The model under review builds one solid part; all positions refer to its coordinate system, in mm. Coordinates: 2 decimals unless noted, no trailing zeros. Write each loop counter-clockwise with the first axis right and the second up, starting at its lowest first coordinate (ties: lowest second). Pieces come first, ordered by that corner, then holes. Notation, with made-up numbers: (38.25, -33) - (45.25, -33) arc R14 cw to (45.25, -29) - close; hole circle Ø6 at (-23.75, -10.5). An arc over 180 degrees is marked (long way). Put each result on its own line as item: value.
from build123d import *

# Parameters (mm, degrees)
BOSS_EXTRUDE1_DEPTH = 914.4
SKETCH2_R           = 6.35
CUT_EXTRUDE1_DEPTH  = 153.4


with BuildPart() as part:
    # Sketch1 → Boss-Extrude1 (new body, symmetric)
    with BuildSketch(Plane.XY):
        with BuildLine():
            Line((0, 0), (0, 152.4))
            Line((0, 152.4), (0.00508, 152.4))
            ThreePointArc((0.00508, 152.4), (6.736679988, 149.611679988), (9.525, 142.88008))
            Line((9.525, 142.88008), (9.525, 22.225))
            ThreePointArc((9.525, 22.225), (13.244743879, 13.244743879), (22.225, 9.525))
            Line((22.225, 9.525), (41.28008, 9.525))
            ThreePointArc((41.28008, 9.525), (48.011679988, 6.736679988), (50.8, 0.00508))
            Line((50.8, 0.00508), (50.8, 0))
            Line((50.8, 0), (0, 0))
        make_face()
    extrude(amount=BOSS_EXTRUDE1_DEPTH, both=True)

    # Sketch2 → Cut-Extrude1 (cut, through all)
    with BuildSketch(Plane.XZ):
        with Locations((25.4, -711.2)):
            Circle(SKETCH2_R)
        with Locations((25.4, -203.2)):
            Circle(SKETCH2_R)
        with Locations((25.4, 203.2)):
            Circle(SKETCH2_R)
        with Locations((25.4, 711.2)):
            Circle(SKETCH2_R)
    extrude(amount=-CUT_EXTRUDE1_DEPTH, mode=Mode.SUBTRACT)


solid = part.part
1. For pin 1 Ø3 at (x, z) = (25, -299) entering from +Y (3 decimals); pin 2 Ø3 at (y, z) = (127, 297.5) entering from +X (3 decimals), all flat-tipped, find the tip position at first contact; note any pin that passes through.
Determined:
pin 1: stops at y = 9.525
pin 2: stops at x = 9.525
2. To check wall thickness, follow probe 1 along Z at (x, y) = (25.4, 5); probe 2 along Y at (x, z) = (22, -556.5); probe 3 along X at (y, z) = (140.5, -86.5) (3 decimals). State the ranges of each line that lie inside material, in increasing order.
Determined:
probe 1: z = -914.4 to -717.55, -704.85 to -209.55, -196.85 to 196.85, 209.55 to 704.85, 717.55 to 914.4
probe 2: y = 0 to 9.53
probe 3: x = 0 to 9.525
3. Consider section B-B on y = 100.5. State the section outline as (x, z) points (3 decimals).
Determined:
outline: (0, -914.4) - (9.525, -914.4) - (9.525, 914.4) - (0, 914.4) - close
4. Consider section A-A on z = 75. State the section outline as (x, y) points (3 decimals), plus the area to 3 significant figures.
Determined:
outline: (0, 0) - (50.8, 0) - (50.8, 0.005) arc R9.52 ccw to (41.28, 9.525) - (22.225, 9.525) arc R12.7 cw to (9.525, 22.225) - (9.525, 142.88) arc R9.52 ccw to (0.005, 152.4) - (0, 152.4) - close
area: 1,840 mm^2
5. The part is to be moulded in two halves that separate along X. For faces 1 (the flat face through (9.525, 83, 13)), 2 (the flat face through (26, 0, 13)), 3 (the flat face through (0, 75, 13)), say which applies: +X half, -X half, draft (parallel to the pull), parting line (faces both ways), or undercut.
Determined:
face 1: +X half
face 2: draft
face 3: -X half
